Source: CAD feature listing. Evaluate the final solid. Frame: model axes, mm. A direction names the side the tool comes from. Give positions to 0.01 mm unless a question says otherwise; leave off trailing zeros. Loops run counter-clockwise (first coordinate to the right, second up) from the corner with the lowest first, then second, coordinate; pieces in that order, holes last. Notation, with made-up numbers: M 45,-4.5 L 74,-4.5 A20 ccw 74,2.5 Z; hole C -3,-35 d6. An arc over 180 degrees is marked long. Answer in a Markdown table with one row per item.
```python
from build123d import *

# Parameters (mm, degrees)
PAD_DEPTH            = 625
SKETCH001_W          = 2.5
SKETCH001_H          = 35.5
POCKET_DEPTH         = 35
BODY_PLACEMENT_ANGLE = 90


with BuildPart() as part:
    # Sketch → Pad (new body)
    with BuildSketch(Plane.XY):
        Polygon((0, 0), (35, 0), (35, -30), (0, -30), (0, -18), (6.5, -18), (6.5, -24.5), (28.5, -24.5), (28.5, -5.5), (6.5, -5.5), (6.5, -12), (0, -12), align=None)
    extrude(amount=PAD_DEPTH)

    # Sketch001 → Pocket (cut)
    with BuildSketch(Plane(origin=(0, 0, 0), x_dir=(0, -1, 0), z_dir=(-1, 0, 0))):
        with Locations((28.850513, 28.757815)):
            Rectangle(SKETCH001_W, SKETCH001_H)
        with Locations((1.206441, 28.56098)):
            Rectangle(SKETCH001_W, SKETCH001_H)
    extrude(amount=-POCKET_DEPTH, mode=Mode.SUBTRACT)


with BuildPart() as part_1:
    # Body placement: moved
    add(part.part.rotate(Axis((0, 0, 0), (0, 0, 1)), BODY_PLACEMENT_ANGLE))


solid = part_1.part
```
Q1. Reachability of faces 4 (the flat face through (5.5, 18, 308)), 5 (the flat face through (2.456, 17, 28)), 6 (the flat face through (0, 17, 5)), 7 (the flat face through (27.601, 17, 29)) from +Z, -Z, +X, -X, +Y, -Y: full face, straight path, thin tool, end or side. Return the list, or none.
Values follow:
| item | result |
|---|---|
| face 4 | +Z, -Z |
| face 5 | -X, +Y, -Y |
| face 6 | +Z, -Z, -X, +Y, -Y |
| face 7 | +X, +Y, -Y |
Q2. Contact query for flat-ended pins moving along their axis: pin 1 Ø4 at (x, y) = (12.5, 9.5) entering from +Z; pin 2 Ø4 at (x, z) = (15.5, 112) entering from -Y. Output: stop coordinate, or through.
Values follow:
| item | result |
|---|---|
| pin 1 | through |
| pin 2 | y = 28.5 |
Q3. Section query A-A (y = 16). Output: boundary loops of the cut face in (x, z).
Values follow:
| item | result |
|---|---|
| outline | M 0,0 L 5.5,0 L 5.5,625 L 0,625 L 0,46.31 L 2.46,46.31 L 2.46,10.81 L 0,10.81 Z; M 24.5,0 L 30,0 L 30,11.01 L 27.6,11.01 L 27.6,46.51 L 30,46.51 L 30,625 L 24.5,625 Z |
Q4. Ray query, probe 1 along Y at (x, z) = (18.5, 377); probe 2 along X at (y, z) = (21.5, 307.5); probe 3 along Y at (x, z) = (12.5, 498.5). Return the intervals inside material, ascending. Write a range as from..to.
Values follow:
| item | result |
|---|---|
| probe 1 | 0..6.5, 28.5..35 |
| probe 2 | 0..5.5, 24.5..30 |
| probe 3 | 28.5..35 |
Q5. Section query B-B (z = 419). Output: boundary loops of the cut face in (x, y).
Values follow:
| item | result |
|---|---|
| outline | M 0,0 L 12,0 L 12,6.5 L 5.5,6.5 L 5.5,28.5 L 24.5,28.5 L 24.5,6.5 L 18,6.5 L 18,0 L 30,0 L 30,35 L 0,35 Z |
Q6. Mould query, pull axis Y, two halves, no side actions, for faces 1 (the flat face through (15, 35, 308)), 2 (the flat face through (24.5, 17, 308)), 3 (the flat face through (30, 18, 5)). Classes: +Y half, -Y half, draft (parallel to the pull), parting line (faces both ways), or undercut.
Values follow:
| item | result |
|---|---|
| face 1 | +Y half |
| face 2 | undercut |
| face 3 | draft |
